Build history of the part. All positions in model axes, mm. A direction names the side the tool comes from. Round coordinates to 2 decimals unless told otherwise and drop trailing zeros. Write each loop counter-clockwise with the first axis right and the second up, starting at its lowest first coordinate (ties: lowest second). Pieces come first, ordered by that corner, then holes. Notation, with made-up numbers: M -8,32.5 L -1,32.5 A26 cw -1,47.5 Z; hole C 79,-32.5 d11. An arc over 180 degrees is marked long. Write item = value, one per line.
from build123d import *

# Parameters (mm, degrees)
F1_R        = 5
F1_R_2      = 3.5
F2_DEPTH    = 30
F4_W        = 1.5
F4_H        = 2.639524132
F5_DEPTH    = 29.5
F6_COUNT    = 4
F8_R        = 3.5
F8_R_2      = 1.25
F9_DEPTH    = 1.5
F10_SIZE2   = 1.49999
F10_SIZE    = 9.99999
F10_2_SIZE2 = 1.49999
F10_2_SIZE  = 9.99999
F10_3_SIZE2 = 1.49999
F10_3_SIZE  = 9.99999
F10_4_SIZE2 = 1.49999
F10_4_SIZE  = 9.99999
F11_SIZE    = 0.5
F12_R       = 0.49999


# Not quite as in the source:
# - a fillet or chamfer is up to 0.001 mm smaller than in the source, because OpenCascade refuses the exact size


with BuildPart() as f2:
    # F1 (on offset) → F2 (new body)
    with BuildSketch(Plane.XY):
        with Locations((-25, 25)):
            Circle(F1_R)
        with Locations((-25, 25)):
            Circle(F1_R_2, mode=Mode.SUBTRACT)
    extrude(amount=-F2_DEPTH)

    # F4 (on offset) → F5 (join)
    with BuildSketch(Plane.XY):
        with Locations((-25, 30.180237934)):
            Rectangle(F4_W, F4_H)
    extrude(amount=-F5_DEPTH)

    # F6: F2 ×4 about axis
    f6_axis = Axis((-25, 25, 0), (0, 0, 1))


with BuildPart() as f2_1:
    add(f2.part)
    for i in range(1, F6_COUNT):
        add(f2.part.rotate(f6_axis, i * 360 / F6_COUNT))

    # F8 (on offset) → F9 (join)
    with BuildSketch(Plane.XY.offset(-30)):
        with Locations((-25, 25)):
            Circle(F8_R)
        with Locations((-25, 25)):
            Circle(F8_R_2, mode=Mode.SUBTRACT)
    extrude(amount=F9_DEPTH)

    # F10 (size 10 and 1.5 in the source; OpenCascade refuses exactly that, so slightly less here)
    f10_edges = [f2_1.edges().sort_by_distance(p)[0] for p in [
        (-25, 18.5, -29.5),
    ]]
    f10_side = f2_1.faces().sort_by_distance((-25, 18.5, -14.75))[0]
    chamfer(f10_edges, length=F10_SIZE, length2=F10_SIZE2, reference=f10_side)

    # F10#2 (size 10 and 1.5 in the source; OpenCascade refuses exactly that, so slightly less here)
    f10_2_edges = [f2_1.edges().sort_by_distance(p)[0] for p in [
        (-18.5, 25, -29.5),
    ]]
    f10_2_side = f2_1.faces().sort_by_distance((-18.5, 25, -14.75))[0]
    chamfer(f10_2_edges, length=F10_2_SIZE, length2=F10_2_SIZE2, reference=f10_2_side)

    # F10#3 (size 10 and 1.5 in the source; OpenCascade refuses exactly that, so slightly less here)
    f10_3_edges = [f2_1.edges().sort_by_distance(p)[0] for p in [
        (-25, 31.5, -29.5),
    ]]
    f10_3_side = f2_1.faces().sort_by_distance((-25, 31.5, -14.75))[0]
    chamfer(f10_3_edges, length=F10_3_SIZE, length2=F10_3_SIZE2, reference=f10_3_side)

    # F10#4 (size 10 and 1.5 in the source; OpenCascade refuses exactly that, so slightly less here)
    f10_4_edges = [f2_1.edges().sort_by_distance(p)[0] for p in [
        (-31.5, 25, -29.5),
    ]]
    f10_4_side = f2_1.faces().sort_by_distance((-31.5, 25, -14.75))[0]
    chamfer(f10_4_edges, length=F10_4_SIZE, length2=F10_4_SIZE2, reference=f10_4_side)

    # F11
    f11_edges = [f2_1.edges().sort_by_distance(p)[0] for p in [
        (-28.5, 25, 0),
        (-26.25, 25, -28.5),
    ]]
    chamfer(f11_edges, length=F11_SIZE)

    # F12 (radius 0.5 in the source; OpenCascade refuses exactly that, so slightly less here)
    f12_edges = [f2_1.edges().sort_by_distance(p)[0] for p in [
        (-30, 25, -30),
    ]]
    fillet(f12_edges, radius=F12_R)


solid = f2_1.part
1. Band-saw the part on D-D (y = 30.75). List the corners of the cut face in (x, z).
Responses:
outline = M -25.75,-24.5 L -24.25,-24.5 L -24.25,0 L -25.75,0 Z
2. Flat gauge pins, fed straight in: pin 1 (2 mm diameter, centred on y = 26, z = -20.5, fed in from -X); pin 2 (1 mm diameter, centred on x = -28.5, z = -27, fed in from -Y); pin 3 (0.5 mm diameter, centred on y = 31, z = -14.5, fed in from -X). Where does each tip first touch, or does it go through?
Responses:
pin_1 = -31.5
pin_2 = 21
pin_3 = -25.75
3. Mould opens along Y. For faces 1 (the face through (-21.66, 26.05, -14.3)), 2 (the face through (-24.25, 31, -11)), 3 (the face through (-25.01, 30.74, -24.57)), 4 (the face through (-27, 24, -28.5)) say: pulls with the +Y half, pulls with the -Y half, needs draft (parallel to the pull), parting line crosses it, or undercut.
Responses:
face_1 = undercut
face_2 = needs draft
face_3 = pulls with the +Y half
face_4 = undercut
4. Tool access for faces 5 (the face through (-23.845, 24.521, -29.507)), 6 (the face through (-19, 24.25, -11)), 7 (the face through (-25.75, 19, -11)), 8 (the face through (-30.74, 24.99, -24.57)), 9 (the face through (-31, 25.75, -11)): list every direction of +Z, -Z, +X, -X, +Y, -Y with a clear straight run to the whole face (end or side of a thin tool).
Responses:
face_5 = +Z, -Z
face_6 = +Z, -Z, +X, -Y
face_7 = +Z, -Z, -X, -Y
face_8 = -Z, -X, +Y, -Y
face_9 = +Z, -Z, -X, +Y
5. Band-saw the part on C-C (z = -16.5). List the corners of the cut face in (x, y), plus the area to 3 significant figures.
Responses:
outline = M -31.5,24.25 L -29.94,24.25 A5 ccw -25.75,20.06 L -25.75,18.5 L -24.25,18.5 L -24.25,20.06 A5 ccw -20.06,24.25 L -18.5,24.25 L -18.5,25.75 L -20.06,25.75 A5 ccw -24.25,29.94 L -24.25,31.5 L -25.75,31.5 L -25.75,29.94 A5 ccw -29.94,25.75 L -31.5,25.75 Z; hole C -25,25 d7
area = 49.2 mm²
6. Probe probe 1 along Z at (x, y) = (-22, 25.5); probe 2 along Y at (x, z) = (-25, -17.25); probe 3 along Y at (x, z) = (-25, -29.5). List the from-to ranges inside material, lowest first.
Responses:
probe_1 = -30 to -28.5
probe_2 = 18.5 to 21.5, 28.5 to 31.5
probe_3 = 20 to 23.75, 26.25 to 30
